Autodesk Fusion 360 part; units mm, degrees
sketch "Sketch1" plane through (0, 0, 0) normal (0, 0, 1) x (1, 0, 0)
  line L0 (7.5, 7.5) -> (-7.5, 7.5)
  line L1 (-7.5, 7.5) -> (-7.5, -7.5)
  line L2 (-7.5, -7.5) -> (7.5, -7.5)
  line L3 (7.5, -7.5) -> (7.5, 7.5)
  line L4 (7.5, 7.5) -> (-7.5, -7.5) construction
  line L5 (-7.5, 7.5) -> (7.5, -7.5) construction
  circle A0 centre (0, 0) radius 1.65
  circle A1 centre (0, 0) radius 3.1
  dimension "d1" = 15
  dimension "d2" = 15
  dimension "d3" = 3.3
  dimension "d9" = 6.2
extrude "Extrude1" add sketch "Sketch1" along normal blind 15 contours L0 L1 L2 L3 | A1
sketch "Sketch2" plane through (0, 7.5, 0) normal (0, 1, 0) x (-1, 0, 0)
  line L0 (-7.5, 0) -> (7.5, 0)
  line L1 (7.5, 0) -> (7.5, 15)
  line L2 (7.5, 15) -> (-7.5, 15)
  line L3 (-7.5, 15) -> (-7.5, 0)
  circle A0 centre (0, 7.5) radius 2.35
  dimension "d6" = 4.7
extrude "Extrude2" cut sketch "Sketch2" against normal blind 4 contours A0
sketch "Sketch3" plane through (0, 0, 15) normal (0, 0, 1) x (1, 0, 0)
  circle A0 centre (0, 0) radius 1.65
  line L0 (7.5, -7.5) -> (7.5, 7.5)
  line L1 (7.5, 7.5) -> (-7.5, 7.5)
  line L2 (-7.5, 7.5) -> (-7.5, -7.5)
  line L3 (-7.5, -7.5) -> (7.5, -7.5)
  circle A1 centre (0, 0) radius 3.1
extrude "Extrude3" cut sketch "Sketch3" against normal blind 13 contours A1
sketch "Sketch4" plane through (-7.5, 0, 0) normal (-1, 0, 0) x (0, 0, 1)
  line L0 (0, 7.5) -> (0, -7.5)
  line L1 (0, -7.5) -> (15, -7.5)
  line L2 (15, -7.5) -> (15, 7.5)
  line L3 (15, 7.5) -> (0, 7.5)
  line L4 (15, 1) -> (12, -2)
  line L5 (0, -7.5) -> (12, -7.5)
  line L6 (15, 1) -> (15, 7.5)
  line L7 (5.15, 3.5) -> (9.85, 3.5)
  line L8 (5.15, 7.5) -> (9.85, 7.5)
  line L9 (12, -4) -> (0, -4)
  line L10 (12, -2) -> (12, -4)
  line L11 (12, -4) -> (12, -7.5)
  dimension "d12" = 12
  dimension "d20" = 3
  dimension "d21" = 3.5
  dimension "d22" = 135
  dimension "d23" = 5.5
extrude "Extrude4" cut sketch "Sketch4" against normal blind 186 contours L1 L2 L4 L10 L11
fillet "Fillet1" radius 0.5 4 edges at (-5.2171, 1, 15) (5.2171, 1, 15) (4.9343, -2, 12) (-4.9343, -2, 12)
fillet "Fillet2" radius 1.5 10 edges at (7.5, 4.3536, 15) (7.5, 1.0158, 14.9619) (7.5, -0.5, 13.5) (7.5, -2.0158, 12.0381) (7.5, -4.8536, 12) (-7.5, 4.3536, 15) (-7.5, 1.0158, 14.9619) (-7.5, -0.5, 13.5) (-7.5, -2.0158, 12.0381) (-7.5, -4.8536, 12)
chamfer "Chamfer2" distance 0.5 angle 45 1 edges at (2.191, 7.5, 8.3498)
chamfer "Chamfer1" distance 0.4 angle 45 1 faces at (0.0411, -5.5485, 0)
chamfer "Chamfer3" distance 0.4 angle 45 1 faces at (2, -7.5, 4.2667)
sketch "Sketch5" plane through (0, -7.5, 0) normal (0, -1, 0) x (1, 0, 0)
  line L0 (7.1, 0.8) -> (7.1, 10.5)
  line L1 (-7.1, 10.5) -> (-7.1, 0.8)
  line L2 (-7.1, 0.8) -> (7.1, 0.8)
  circle A0 centre (0, 8) radius 2
  line L3 (-7.1, 0) -> (7.1, 0)
  arc A1 (7.1, 10.5) -> (6, 11.6) centre (6, 10.5) ccw
  line L4 (6, 11.6) -> (-6, 11.6)
  arc A2 (-6, 11.6) -> (-7.1, 10.5) centre (-6, 10.5) ccw
  line L5 (6, 12) -> (-6, 12)
  dimension "d28" = 8
  dimension "d29" = 4
  dimension "d34" = 4
extrude "Extrude5" cut sketch "Sketch5" against normal blind 2 contours A0
chamfer "Chamfer4" distance 0.4 angle 45 6 edges at (-1.8647, -7.5, 8.7232) (7.5, 7.5, 6.95) (7.0607, 7.5, 14.5607) (0, 7.5, 15) (-7.0607, 7.5, 14.5607) (-7.5, 7.5, 6.95)
sketch "Sketch6" plane through (0, 0, 0) normal (0, 0, -1) x (-1, 0, 0)
  circle A0 centre (0, 0) radius 2.05
  line L0 (-7.1, 7.1) -> (-7.1, -7.1)
  line L1 (-7.1, -7.1) -> (7.1, -7.1)
  line L2 (7.1, -7.1) -> (7.1, 7.1)
  line L3 (7.1, 7.1) -> (-7.1, 7.1)
  line L4 (-3.25, 6.7) -> (3.25, 6.7)
  line L5 (3.25, 6.7) -> (3.25, 3.7)
  line L6 (3.25, 3.7) -> (-3.25, 3.7)
  line L7 (-3.25, 3.7) -> (-3.25, 6.7)
  line L8 (-7.5, 7.1) -> (-7.5, -7.1)
  line L9 (7.1, 7.5) -> (-7.1, 7.5)
  dimension "d35" = 6.5
  dimension "d36" = 3
  dimension "d37" = 4.25
  dimension "d38" = 0.8
extrude "Extrude6" cut sketch "Sketch6" against normal blind 2 contours L4 L5 L6 L7
chamfer "Chamfer5" distance 0.25 angle 45 4 edges at (-3.25, 5.2, 0) (0, 6.7, 0) (0, 3.7, 0) (3.25, 5.2, 0)
equation "d10 = -15 mm + 2 mm"
CAD build for the part. Positions are in the model's coordinates, mm. A direction names the side the tool comes from. Give positions to 0.01 mm unless a question says otherwise; leave off trailing zeros. Order: outer loops, then holes, each group sorted by start corner. A loop starts at its lowest first (then second) coordinate and runs counter-clockwise, first axis right, second up.
(1) Saw through at C-C, the plane y = 6. Give the cut face in (x, z).
(2) Mould opens along X. For faces 5 (the flat face through (-3.25, 5, 1)), 6 (the flat face through (0, 3.7, 1)), 7 (the flat face through (0, -5, 12)), 8 (the conical face through (6.88, -7.34, 11.4)) say: released by +X, released by -X, zero draft, split by the parting line, or undercut.
(3) Flat gauge pins, fed straight in: pin 1 (2.5 mm diameter, centred on x = -0.5, z = 7.5, fed in from +Y); pin 2 (3.5 mm diameter, centred on x = -0.5, y = 4.5, fed in from -Z); pin 3 (4.5 mm diameter, centred on x = 0, z = 8, fed in from +Y); pin 4 (1.5 mm diameter, centred on x = -1.5, y = -1.5, fed in from +Z). Where does each tip first touch, or does it go through?
(4) Saw through at B-B, the plane z = 1.5. Give the cut face in (x, y), then the cut area to 3 significant figures.
(5) Tool access for faces 1 (the cylindrical face through (-7.05, -4.69, 11.57)), 2 (the cylindrical face through (0, -6, 10)), 3 (the cylindrical face through (-1.216, -1.115, 1.189)), 4 (the flat face through (0, 6.7, 1)): list every direction of +Z, -Z, +X, -X, +Y, -Y with a clear straight run to the whole face (end or side of a thin tool).
(6) Drill centre lines: L1, parallel to Z at x = 0, y = 4.2; L2, parallel to X at y = 0, z = 9; L3, parallel to X at y = -1.5, z = 10.5. Where is each one in solid material? Low to high.
(7) Saw through at A-A, the plane y = -6. Give the cut face in (x, z).
(8) Saw through at D-D, the plane y = 2.5. Give the cut face in (x, z), then the cut area to 3 significant figures.
Results found:
1. outline: (-7.5, 0.4) - (-7.1, 0) - (-3.5, 0) - (-3.25, 0.25) - (-3.25, 2) - (3.25, 2) - (3.25, 0.25) - (3.5, 0) - (7.1, 0) - (7.5, 0.4) - (7.5, 13.5) arc R1.5 ccw to (6, 15) - (-6, 15) arc R1.5 ccw to (-7.5, 13.5) - close; hole circle Ø4.7 at (0, 7.5)
2. face 5: undercut
2. face 6: undercut
2. face 7: zero draft
2. face 8: released by +X
3. pin 1: stops at y = 3.5
3. pin 2: stops at z = 0
3. pin 3: stops at y = 7.4
3. pin 4: stops at z = 2
4. outline: (-7.5, -7.1) - (-7.1, -7.5) - (7.1, -7.5) - (7.5, -7.1) - (7.5, 7.1) - (7.1, 7.5) - (-7.1, 7.5) - (-7.5, 7.1) - close; hole (-3.25, 3.7) - (3.25, 3.7) - (3.25, 6.7) - (-3.25, 6.7) - close; hole circle Ø3.3 at (0, 0)
4. area: 197 mm2
5. face 1: +Z, -X, -Y
5. face 2: -Y
5. face 3: +Z, -Z
5. face 4: -Z
6. L1: z = 2 to 5.15, 9.85 to 15
6. L2: x = -7.5 to -3.1, 3.1 to 7.5
6. L3: x = -7.5 to -2.71, 2.71 to 7.5
7. outline: (-7.5, 0.4) - (-7.1, 0) - (7.1, 0) - (7.5, 0.4) - (7.5, 10.5) arc R1.5 ccw to (6, 12) - (-6, 12) arc R1.5 ccw to (-7.5, 10.5) - close; hole circle Ø4 at (0, 8)
8. outline: (-7.5, 0.4) - (-7.1, 0) - (7.1, 0) - (7.5, 0.4) - (7.5, 13.5) arc R1.5 ccw to (6, 15) - (1.83, 15) - (1.83, 2) - (-1.83, 2) - (-1.83, 15) - (-6, 15) arc R1.5 ccw to (-7.5, 13.5) - close
8. area: 176 mm2
